The listing builds one solid part. Answer for the finished solid, in the listing's coordinates (mm). Face numbers are marked on the shaded views. A direction names the side the tool comes from. Give positions to 0.01 mm unless a question says otherwise; leave off trailing zeros. Write each loop counter-clockwise with the first axis right and the second up, starting at its lowest first coordinate (ties: lowest second). Pieces come first, ordered by that corner, then holes. Notation, with made-up numbers: M -31.5,-13.5 L 1.5,-13.5 A15 ccw 1.5,-6.5 Z; hole C 79,-35.5 d9. An arc over 180 degrees is marked long. Answer as a JSON object with one key per item and string values.
```python
from build123d import *

# Parameters (mm, degrees)
BOSS_EXTRUDE1_DEPTH  = 3
BALL1_REVOLVED_ANGLE = 180
BOSS_EXTRUDE3_DEPTH  = 3


with BuildPart() as part:
    # Sketch1 → Boss-Extrude1 (new body)
    with BuildSketch(Plane.XY):
        Polygon((10, 0), (30, 0), (30, 3), (27, 3), (-27, 3), (-30, 3), (-30, 0), (-10, 0), (-10, -20), (-30, -20), (-30, -23), (-27, -23), (27, -23), (30, -23), (30, -20), (10, -20), align=None)
    extrude(amount=BOSS_EXTRUDE1_DEPTH)

    # ball1 → ball1_revolved (revolve)
    with BuildSketch(Plane(origin=(0, 3, 0), x_dir=(1, 0, 0), z_dir=(0, 1, 0))):
        with BuildLine():
            Line((30, -1.5), (27, -1.5))
            ThreePointArc((27, -1.5), (28.5, 0), (30, -1.5))
        make_face()
    revolve(axis=Axis((30, 3, 1.5), (1, 0, 0)), revolution_arc=BALL1_REVOLVED_ANGLE)

    # Sketch8 → Boss-Extrude3 (add)
    with BuildSketch(Plane(origin=(0, 0, 0), x_dir=(-1, 0, 0), z_dir=(0, 0, -1))):
        Polygon((-5.757359313, 0), (-10, 0), (-10, -4.242640687), (-4.242640687, -10), (0, -5.757359313), align=None)
        Polygon((5.757359313, 0), (0, -5.757359313), (4.242640687, -10), (10, -4.242640687), (10, 0), align=None)
        Polygon((4.242640687, -10), (0, -5.757359313), (-4.242640687, -10), (0, -14.242640687), align=None)
        Polygon((10, -15.757359313), (4.242640687, -10), (0, -14.242640687), (5.757359313, -20), (10, -20), align=None)
        Polygon((0, -14.242640687), (-4.242640687, -10), (-10, -15.757359313), (-10, -20), (-5.757359313, -20), align=None)
    extrude(amount=BOSS_EXTRUDE3_DEPTH)

    # Sketch5 → Revolve4 (revolve)
    with BuildSketch(Plane.XZ.offset(23)):
        with BuildLine():
            ThreePointArc((28.5, 3), (27.439339828, 2.560660172), (27, 1.5))
            Line((27, 1.5), (30, 1.5))
            ThreePointArc((30, 1.5), (29.560660172, 2.560660172), (28.5, 3))
        make_face()
        with BuildLine():
            ThreePointArc((-27, 1.5), (-28.5, 3), (-30, 1.5))
            Line((-30, 1.5), (-27, 1.5))
        make_face()
    revolve(axis=Axis((-30, -23, 1.5), (1, 0, 0)))

    # ball2 → Revolve5 (revolve)
    with BuildSketch(Plane(origin=(0, 3, 0), x_dir=(1, 0, 0), z_dir=(0, 1, 0))):
        with BuildLine():
            Line((-30, -1.5), (-27, -1.5))
            ThreePointArc((-27, -1.5), (-28.5, -3), (-30, -1.5))
        make_face()
    revolve(axis=Axis((-30, 3, 1.5), (1, 0, 0)))


solid = part.part
```
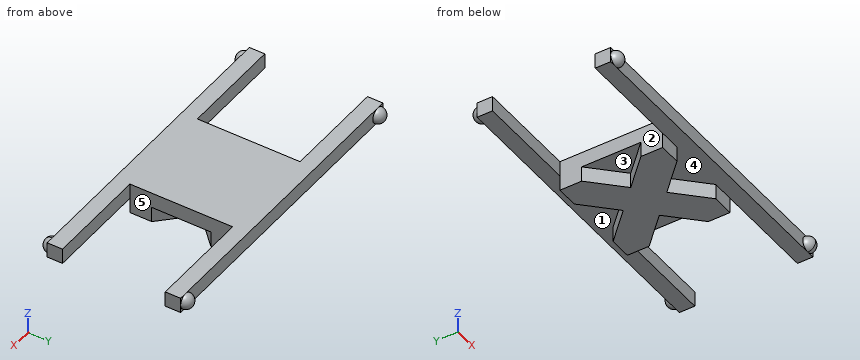
1. A cutting plane is placed at C-C, the plane x = -2. Give the vertices of the cut face in (y, z), plus the area to 3 significant figures.
Verdict:
{"outline": "M -23,0 L -16.24,0 L -16.24,-3 L -3.76,-3 L -3.76,0 L 3,0 L 3,3 L -23,3 Z", "area": "115 mm2"}
2. A cutting plane is placed at A-A, the plane x = 12. Give the vertices of the cut face in (y, z).
Verdict:
{"outline": "M -23,0 L -20,0 L -20,3 L -23,3 Z; M 0,0 L 3,0 L 3,3 L 0,3 Z"}
3. Consider line 1 along Y through (x, z) = (-23.5, 2.5); line 2 along X through (y, z) = (-15.75, 0.5); line 3 along Y through (x, z) = (7, 1.75). Determine where each line is inside the solid, lowest interval first.
Verdict:
{"line 1": "y = -23 to -20, 0 to 3", "line 2": "x = -10 to 10", "line 3": "y = -23 to 3"}
4. A cutting plane is placed at B-B, the plane z = -1.5. Give the vertices of the cut face in (x, y), plus the area to 3 significant figures.
Verdict:
{"outline": "M -10,-20 L -5.76,-20 L 0,-14.24 L 5.76,-20 L 10,-20 L 10,-15.76 L 4.24,-10 L 10,-4.24 L 10,0 L 5.76,0 L 0,-5.76 L -5.76,0 L -10,0 L -10,-4.24 L -4.24,-10 L -10,-15.76 Z", "area": "267 mm2"}
5. A cutting plane is placed at D-D, the plane y = -8.25. Give the vertices of the cut face in (x, z), plus the area to 3 significant figures.
Verdict:
{"outline": "M -10,0 L -5.99,0 L -5.99,-3 L 5.99,-3 L 5.99,0 L 10,0 L 10,3 L -10,3 Z", "area": "96.0 mm2"}
6. The mould has two halves that part along Y. Classify the marked faces 1 and 2: released by +Y, released by -Y, zero draft, split by the parting line, or undercut.
Verdict:
{"face 1": "zero draft", "face 2": "undercut"}
7. For the marked faces 3, 4 and 5, determine the directions among +Z, -Z, +X, -X, +Y, -Y from which every point of the face is accessible in a straight line to the end or side of a thin tool.
Verdict:
{"face 3": "-Z, -X", "face 4": "-Z, -Y", "face 5": "+Z, -Z, +X"}
8. Flat-ended cylindrical pins translate along their axes: pin 1 (3 mm diameter, centred on y = -3.5, z = 1.5, fed in from +X); pin 2 (1.5 mm diameter, centred on y = -8.5, z = 0.5, fed in from -X); pin 3 (1.5 mm diameter, centred on x = 8, z = 1.5, fed in from +Y). Find the tip coordinate at first contact, or state that the pin passes through.
Verdict:
{"pin 1": "stops at x = 10", "pin 2": "stops at x = -10", "pin 3": "stops at y = 3"}
